Part print with two shaded views. Sizes in mm from the minimum x, y, z corner. A direction names the side the tool comes from. Give positions to 0.01 mm unless a question says otherwise; leave off trailing zeros. Order: outer loops, then holes, each group sorted by start corner. A loop starts at its lowest first (then second) coordinate and runs counter-clockwise, first axis right, second up. Notation, with made-up numbers: (21.5, 43.5) -> (65.5, 43.5) arc R15 ccw to (65.5, 66.5) -> close; hole circle Ø10 at (24, -34.5). An arc over 180 degrees is marked (long way). Write item = value, one per line. Start each with the question number.
Item 1: Band-saw the part on A-A on x = 15.5. Write the cut outline in (y, z), plus the area to 3 significant figures.
Item 2: Drill centre lines: line 1 along Y through (x, z) = (44, 2.85); line 2 along X through (y, z) = (30.5, 3.35); line 3 along Y through (x, z) = (4, 4.25). Where is each one in solid material? Low to high.
Item 3: Tool access for the marked faces 1 and 2: list every direction of +Z, -Z, +X, -X, +Y, -Y with a clear straight run to the whole face (end or side of a thin tool).
Item 4: Band-saw the part on B-B on y = 16.5. Write the cut outline in (x, z).
Item 5: Flat gauge pins, fed straight in: P1, Ø2, axis at y = 33.5, z = 1, coming from the +X side; P2, Ø1.5, axis at x = 32.5, z = 4.5, coming from the +Y side; P3, Ø2, axis at x = 39, z = 1, coming from the +Y side. Where does each tip first touch, or does it go through?
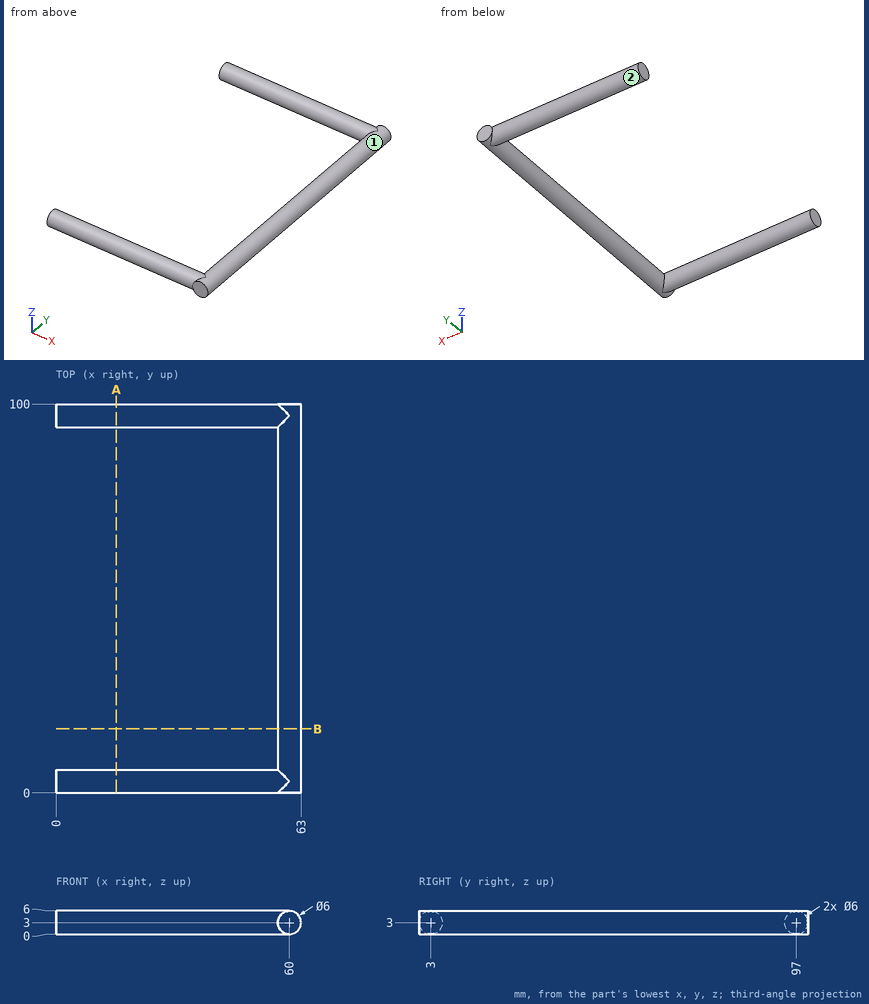
Values found:
q1.outline = circle Ø6 at (3, 3); circle Ø6 at (97, 3)
q1.area = 56.5 mm^2
q2.line_1 = 0 to 6, 94 to 100
q2.line_2 = 57.02 to 62.98
q2.line_3 = 0.27 to 5.73, 94.27 to 99.73
q3.face_1 = none
q3.face_2 = -X
q4.outline = circle Ø6 at (60, 3)
q5.P1 = 62.83
q5.P2 = 99.9
q5.P3 = 99.83
